Part model, mm, in its own coordinate system. A direction names the side the tool comes from. Give positions to 0.01 mm unless a question says otherwise; leave off trailing zeros. Write each loop counter-clockwise with the first axis right and the second up, starting at its lowest first coordinate (ties: lowest second). Pieces come first, ordered by that corner, then holes. Notation, with made-up numbers: (56.25, -36) - (68.25, -36) arc R8 cw to (68.25, -21) - close; hole circle Ø9 at (15.25, 47). An arc over 180 degrees is marked (long way). Answer in a Markdown table with one row per item. Add a question column.
1. Pull direction Y, two halves, no side cores. Call faces 3 (the flat face through (13.43, 15, -8.98)), 4 (the flat face through (13.43, 0, -8.98)), 5 (the cylindrical face through (6.57, 8.36, 16.81)): released by +Y, released by -Y, zero draft, split by the parting line, or undercut.
2. Band-saw the part on C-C on y = 7.5. Write the cut outline in (x, z).
3. Band-saw the part on D-D on z = 9. Write the cut outline in (x, y), plus the area to 3 significant figures.
4. Probe line 1 along Y through (x, z) = (-17, 0); line 2 along X through (y, z) = (11.5, 0); line 3 along Z through (x, y) = (-8, 9). List the from-to ranges inside material, lowest first.
5. Which spindle directions (+Z, -Z, +X, -X, +Y, -Y) get a long thin tool onto all of the face, cutting with end or side? Do faces 1 (the cylindrical face through (11.276, 8.356, -14.093)), 2 (the cylindrical face through (-17.841, 8.356, -2.718)). Say none if no direction does.
6. Band-saw the part on A-A on z = 0. Write the cut outline in (x, y).
7. Band-saw the part on B-B on x = -7. Write the cut outline in (y, z) (1 decimal).
8. Drop flat-ended pins along their axis: pin 1 Ø2 at (x, z) = (9.5, -10.5) entering from -Y; pin 2 Ø8 at (y, z) = (3, 0.5) entering from +X; pin 3 Ø3 at (x, y) = (8.5, 5.5) entering from +Z (3 decimals); pin 4 Ø8 at (y, z) = (9, 4.5) entering from -X. Give the stop position or say it passes through.
```python
from build123d import *

# Parameters (mm, degrees)
CROQUIS1_R              = 20
CROQUIS1_R_2            = 16
SALIENTE_EXTRUIR1_DEPTH = 15
CROQUIS3_R              = 2.85
CORTAR_EXTRUIR1_DEPTH   = 33.015621187
CROQUIS7_R              = 2.85
CORTAR_EXTRUIR3_DEPTH   = 33.015621359
CROQUIS9_R              = 2.85
CORTAR_EXTRUIR5_DEPTH   = 33.015621359


with BuildPart() as part:
    # Croquis1 → Saliente-Extruir1 (new body)
    with BuildSketch(Plane(origin=(0, 0, 0), x_dir=(1, 0, 0), z_dir=(0, 1, 0))):
        with Locations(Location((0, 0, 0), (0, 0, 270))):
            Circle(CROQUIS1_R)
        with Locations(Location((0, 0, 0), (0, 0, 270))):
            Circle(CROQUIS1_R_2, mode=Mode.SUBTRACT)
    extrude(amount=SALIENTE_EXTRUIR1_DEPTH)

    # Croquis3 → Cortar-Extruir1 (cut, through all)
    with BuildSketch(Plane(origin=(0, 0, 0), x_dir=(0, 0, -1), z_dir=(1, 0, 0))):
        with Locations((0, 7.5)):
            Circle(CROQUIS3_R)
    extrude(amount=-CORTAR_EXTRUIR1_DEPTH, mode=Mode.SUBTRACT)

    # Croquis7 → Cortar-Extruir3 (cut, through all)
    with BuildSketch(Plane(origin=(0, 0, 0), x_dir=(0.8660254037844363, 0, 0.500000000000004), z_dir=(-0.5000000000000041, 0, 0.8660254037844364))):
        with Locations((0, 7.5)):
            Circle(CROQUIS7_R)
    extrude(amount=-CORTAR_EXTRUIR3_DEPTH, mode=Mode.SUBTRACT)

    # Croquis9 → Cortar-Extruir5 (cut, through all)
    with BuildSketch(Plane(origin=(0, 0, 0), x_dir=(-0.8660254037844434, 0, 0.499999999999992), z_dir=(-0.499999999999992, 0, -0.8660254037844434))):
        with Locations((0, 7.5)):
            Circle(CROQUIS9_R)
    extrude(amount=-CORTAR_EXTRUIR5_DEPTH, mode=Mode.SUBTRACT)


solid = part.part
```
Values:
| question | item | result |
|---|---|---|
| 1 | face 3 | released by +Y |
| 1 | face 4 | released by -Y |
| 1 | face 5 | undercut |
| 2 | outline | (-19.8, -2.85) arc R20 ccw to (7.43, -18.57) - (5.4, -15.06) arc R16 cw to (-15.74, -2.85) - close; (-19.8, 2.85) - (-15.74, 2.85) arc R16 cw to (5.4, 15.06) - (7.43, 18.57) arc R20 ccw to start; (10.34, -12.21) - (12.37, -15.72) arc R20 ccw to (12.37, 15.72) - (10.34, 12.21) arc R16 cw to start |
| 3 | outline | (-17.86, 0) - (-13.23, 0) - (-13.23, 15) - (-17.86, 15) - close; (13.23, 0) - (17.86, 0) - (17.86, 15) - (13.23, 15) - close |
| 3 | area | 139 mm² |
| 4 | line 1 | y = 0 to 4.65, 10.35 to 15 |
| 4 | line 2 | x = -20 to -16, 16 to 20 |
| 4 | line 3 | z = -18.33 to -13.86, 13.86 to 18.33 |
| 5 | face 1 | none |
| 5 | face 2 | -X |
| 6 | outline | (-20, 0) - (-16, 0) - (-16, 4.65) - (-20, 4.65) - close; (-20, 10.35) - (-16, 10.35) - (-16, 15) - (-20, 15) - close; (16, 0) - (20, 0) - (20, 15) - (16, 15) - close |
| 7 | outline | (0, -18.7) - (15, -18.7) - (15, -14.4) - (0, -14.4) - close; (0, 14.4) - (15, 14.4) - (15, 18.7) - (0, 18.7) - close |
| 8 | pin 1 | passes through |
| 8 | pin 2 | stops at x = 20 |
| 8 | pin 3 | stops at z = 18.735 |
| 8 | pin 4 | stops at x = -19.99 |
